Could you check a few things on this model? Use its own coordinates, in mm. Face numbers are marked on the shaded views. A direction names the side the tool comes from. Give positions to 0.01 mm unless a question says otherwise; leave off trailing zeros. Order: outer loops, then holes, each group sorted by start corner. A loop starts at its lowest first (then second) coordinate and runs counter-clockwise, first axis right, second up. Notation, with made-up numbers: (65, 87.25) -> (81, 87.25) arc R21 cw to (81, 102.25) -> close; hole circle Ø11 at (69.25, 40.25). An arc over 180 degrees is marked (long way). One line per item, written item: value.
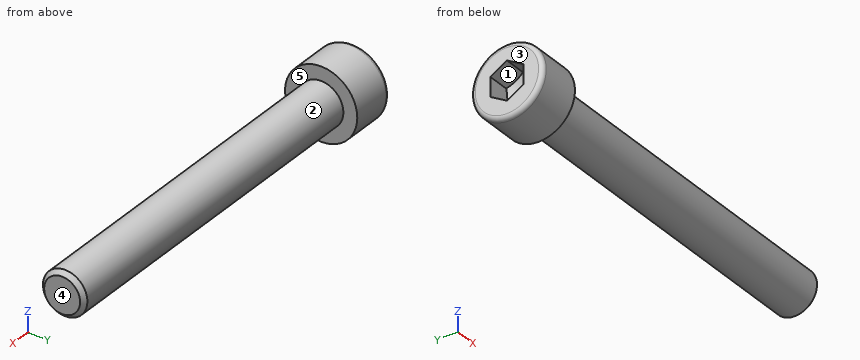
Autodesk Inventor part; units mm, degrees
ref_plane "Work Plane1" through (29, 0, 0) normal (0, -1, 0) x (1, 0, 0)
ref_plane "YZ Plane" through (0, 0, 0) normal (1, 0, 0) x (0, 1, 0)
ref_plane "XZ Plane" through (0, 0, 0) normal (0, 1, 0) x (-1, 0, 0)
sketch "Sketch1" plane through (0, 0, 0) normal (0, 0, 1) x (1, 0, 0)
  line L0 (-2, 0) -> (65, 0)
  line L1 (65, 0) -> (65, 4)
  line L2 (65, 4) -> (37, 4)
  line L3 (37, 4) -> (36.2331, 4)
  line L4 (36.2331, 4) -> (0, 4)
  line L5 (0, 4) -> (0, 6.5)
  line L6 (0, 6.5) -> (-8, 6.5)
  line L7 (-8, 6.5) -> (-8, 3.4641)
  line L8 (-8, 3.4641) -> (-4, 3.4641)
  line L9 (-4, 3.4641) -> (-2, 0)
  line L10 (-15.3, 0) -> (86.9, 0)
  line L11 (0, -0.65) -> (0, 8.45)
  line L12 (37, 4) -> (0, 4) construction
  dimension "d1" = 28
  dimension "d2" = 0.7669
  dimension "d3" = 8
  dimension "d4" = 4
  dimension "d5" = 60
  dimension "d6" = 8
  dimension "d7" = 8
  dimension "d8" = 6.9282
  dimension "d9" = 13
  dimension "d26" = 65
revolve "Body" add sketch "Sketch1" angle 360 about axis through (-2, 0, 0) along (1, 0, 0)
sketch "Sketch2" plane through (-8, 0, 0) normal (-1, 0, 0) x (0, 0, 1)
  circle A0 centre (0, 0) radius 3.4641
  line L0 (0, -7.8) -> (0, 10.4)
  line L1 (-7.8, 0) -> (10.4, 0)
  line L2 (3.4641, 0) -> (1.7321, -3)
  line L3 (1.7321, -3) -> (-1.7321, -3)
  line L4 (-1.7321, -3) -> (-3.4641, 0)
  line L5 (-3.4641, 0) -> (-1.7321, 3)
  line L6 (-1.7321, 3) -> (1.7321, 3)
  line L7 (1.7321, 3) -> (3.4641, 0)
extrude "Slot" add sketch "Sketch2" against normal up to next contours L7 A0 | A0 L2 | L6 L0 A0 | A0 L0 L3 | L0 L6 A0 | A0 L3 L0 | L4 A0 | A0 L5
fillet "Fillet1" radius 0.8 1 edges at (-8, -6.5, 0)
thread "Thread"
chamfer "Chamfer1" distance 0.7668 distance2 0.7668 1 edges at (65, -4, 0) measured on face at (65, -1.1806, -1.575)
ref_plane "Work Plane1" through (29, 0, 0) normal (0, -1, 0) x (1, 0, 0)
equation "\"d1\" = GEL"
equation "\"d3\" = KOH"
equation "\"d4\" = INTI"
equation "\"d6\" = GD"
equation "\"d7\" = BDM"
equation "\"d8\" = 1.1547 * SW"
equation "\"d9\" = KOD"
equation "\"d26\" = NLG"
equation "\"d17\" = RR"
equation "\"d13\" = GEL"
equation "\"d15\" = -0.5 * SPD + 0.5 * GD"
equation "\"d16\" = GUL"
equation "\"GD\" = 8"
equation "\"NLG\" = 65"
equation "\"GEL\" = 28"
equation "\"KOD\" = 13"
equation "\"KOH\" = 8"
equation "\"INTI\" = 4"
equation "\"GAL\" = 0.61345 * PTC"
equation "\"GUL\" = 0.61345 * PTC"
equation "\"BDM\" = NND"
equation "\"SW\" = 6"
equation "\"RR\" = 0.8"
equation "\"SPD\" = NND - 1.2269 * PTC"
equation "\"TOA\" = 30deg"
equation "\"GD1\" = THREADDIA - 1.2269 * PTC"
equation "\"THREADDIA\" = 8"
equation "\"FAWI\" = 45deg"
equation "\"PTC\" = 1.25"
equation "\"NND\" = 8"
equation "\"E0\" = 1.155 * SW"
properties part number "100021" material "Steel, Mild"
1) We'd pull the mould along Z, two halves only. Please class the marked faces 1, 2 and 3: +Z half, -Z half, draft (parallel to the pull), parting line (faces both ways), or undercut.
Answer below:
face 1: undercut
face 2: parting line
face 3: draft
2) For the marked faces 4 and 5, which set-ups out of +Z, -Z, +X, -X, +Y, -Y let a thin tool reach every point of the face, with its end or its side?
Answer below:
face 4: +Z, -Z, +X, +Y, -Y
face 5: +X
3) For P1, Ø1, axis at x = 33.5, z = 0.5, coming from the +Y side; P2, Ø2, axis at x = 52, z = -4.5, coming from the -Y side; P3, Ø1, axis at x = 16, z = 1.5, coming from the -Y side, each with a flat end and sliding along its axis, tell me the tip position at first contact or that it passes through.
Answer below:
P1: stops at y = 4
P2: stops at y = -1.94
P3: stops at y = -3.87
4) If I drill on line 1 along X through (y, z) = (3, -4); line 2 along Y through (x, z) = (37, 0.25); line 3 along Y through (x, z) = (11.5, 3.5), over which ranges is the centre line in solid material (lowest first)?
Answer below:
line 1: x = -8 to 0
line 2: y = -3.99 to 3.99
line 3: y = -1.94 to 1.94
5) Suppose I cut it at A-A, the plane x = 23. Write out the boundary of the cut face in (y, z).
Answer below:
outline: circle Ø8 at (0, 0)
